The listing builds one solid part. Answer for the finished solid, in the listing's coordinates (mm). A direction names the side the tool comes from. Give positions to 0.01 mm unless a question says otherwise; leave off trailing zeros. Write each loop counter-clockwise with the first axis right and the second up, starting at its lowest first coordinate (ties: lowest second). Pieces come first, ordered by that corner, then holes. Notation, with made-up numbers: (70, -15.75) - (99, -15.75) arc R10 ccw to (99, 0.25) - close; hole circle Ø1 at (80, 60.25). An arc over 180 degrees is marked (long way). One line per item, written item: value. Start each with the question number.
Autodesk Inventor part; units mm, degrees
ref_plane "to_body_XY" through (0, 0, 0) normal (0, -1, 0) x (1, 0, 0)
ref_plane "to_body_YZ" through (0, 0, 0) normal (1, 0, 0) x (0, 0, 1)
ref_plane "to_body_ZX" through (0, 0, 0) normal (0, 0, 1) x (0, -1, 0)
sketch "Sketch_1" plane through (0, 0.508, 0) normal (0, 1, 0) x (1, 0, 0)
  line L0 (-4.445, 8.382) -> (-4.445, -8.382)
  line L1 (-4.445, -8.382) -> (4.445, -8.382)
  line L2 (4.445, -8.382) -> (4.445, 8.382)
  line L3 (4.445, 8.382) -> (-4.445, 8.382)
extrude "Extrusion1" add sketch "Sketch_1" against normal blind 0.254
sketch "Sketch_2" plane through (-2.4892, 0, 0) normal (1, 0, 0) x (0, 0, -1)
  line L0 (-7.3787, -7.62) -> (-6.9342, -8.255)
  line L1 (-6.9342, -8.255) -> (-3.0734, -8.255)
  line L2 (-3.0734, -8.255) -> (-2.6289, -7.62)
  line L3 (-2.6289, -7.62) -> (-2.6289, 0.508)
  line L4 (-2.6289, 0.508) -> (-7.3787, 0.508)
  line L5 (-7.3787, 0.508) -> (-7.3787, -7.62)
  arc A0 (-4.2207, -5.6252) -> (-5.7869, -5.6252) centre (-5.0038, -4.7752) ccw
  arc A1 (-5.7869, -5.6252) -> (-4.2207, -5.6252) centre (-5.0038, -5.461) ccw
extrude "Extrusion2" add sketch "Sketch_2" along normal mid plane 0.7874
sketch "Sketch_3" plane through (2.4892, 0, 0) normal (1, 0, 0) x (0, 0, -1)
  line L0 (-7.3787, -7.62) -> (-6.9342, -8.255)
  line L1 (-6.9342, -8.255) -> (-3.0734, -8.255)
  line L2 (-3.0734, -8.255) -> (-2.6289, -7.62)
  line L3 (-2.6289, -7.62) -> (-2.6289, 0.508)
  line L4 (-2.6289, 0.508) -> (-7.3787, 0.508)
  line L5 (-7.3787, 0.508) -> (-7.3787, -7.62)
  arc A0 (-4.2207, -5.6252) -> (-5.7869, -5.6252) centre (-5.0038, -4.7752) ccw
  arc A1 (-5.7869, -5.6252) -> (-4.2207, -5.6252) centre (-5.0038, -5.461) ccw
extrude "Extrusion3" add sketch "Sketch_3" along normal mid plane 0.7874
sketch "Sketch_4" plane through (-3.9878, 0, 0) normal (1, 0, 0) x (0, 0, -1)
  line L0 (0.9779, -0.3048) -> (0.9779, -1.016)
  line L1 (0.9779, -1.016) -> (1.6129, -1.016)
  line L2 (1.6129, -1.016) -> (1.6129, -7.62)
  line L3 (1.6129, -7.62) -> (2.0574, -8.255)
  line L4 (2.0574, -8.255) -> (5.9182, -8.255)
  line L5 (5.9182, -8.255) -> (6.3627, -7.62)
  line L6 (6.3627, -7.62) -> (6.3627, 0.508)
  line L7 (6.3627, 0.508) -> (1.6129, 0.508)
  line L8 (1.6129, 0.508) -> (1.6129, -0.3048)
  line L9 (1.6129, -0.3048) -> (0.9779, -0.3048)
  arc A0 (4.7709, -5.6252) -> (3.2047, -5.6252) centre (3.9878, -4.7752) ccw
  arc A1 (3.2047, -5.6252) -> (4.7709, -5.6252) centre (3.9878, -5.461) ccw
extrude "Extrusion4" add sketch "Sketch_4" along normal mid plane 0.7874
sketch "Sketch_5" plane through (3.9878, 0, 0) normal (1, 0, 0) x (0, 0, -1)
  line L0 (0.9779, -0.3048) -> (0.9779, -1.016)
  line L1 (0.9779, -1.016) -> (1.6129, -1.016)
  line L2 (1.6129, -1.016) -> (1.6129, -7.62)
  line L3 (1.6129, -7.62) -> (2.0574, -8.255)
  line L4 (2.0574, -8.255) -> (5.9182, -8.255)
  line L5 (5.9182, -8.255) -> (6.3627, -7.62)
  line L6 (6.3627, -7.62) -> (6.3627, 0.508)
  line L7 (6.3627, 0.508) -> (1.6129, 0.508)
  line L8 (1.6129, 0.508) -> (1.6129, -0.3048)
  line L9 (1.6129, -0.3048) -> (0.9779, -0.3048)
  arc A0 (4.7709, -5.6252) -> (3.2047, -5.6252) centre (3.9878, -4.7752) ccw
  arc A1 (3.2047, -5.6252) -> (4.7709, -5.6252) centre (3.9878, -5.461) ccw
extrude "Extrusion5" add sketch "Sketch_5" along normal mid plane 0.7874
sketch "Sketch_6" plane through (0, 0, 0) normal (0, 0, 1) x (1, 0, 0)
  line L0 (-5.08, -8.636) -> (5.08, -8.636)
  line L1 (5.08, -8.636) -> (5.08, 0)
  line L2 (5.08, 0) -> (4.3815, 0)
  line L3 (4.3815, 0) -> (4.3815, -7.62)
  line L4 (4.3815, -7.62) -> (4.2545, -8.255)
  line L5 (4.2545, -8.255) -> (3.7211, -8.255)
  line L6 (3.7211, -8.255) -> (3.5941, -7.62)
  line L7 (3.5941, -7.62) -> (3.5941, 0)
  line L8 (3.5941, 0) -> (2.8829, 0)
  line L9 (2.8829, 0) -> (2.8829, -7.62)
  line L10 (2.8829, -7.62) -> (2.7559, -8.255)
  line L11 (2.7559, -8.255) -> (2.2225, -8.255)
  line L12 (2.2225, -8.255) -> (2.0955, -7.62)
  line L13 (2.0955, -7.62) -> (2.0955, 0)
  line L14 (2.0955, 0) -> (-2.0955, 0)
  line L15 (-2.0955, 0) -> (-2.0955, -7.62)
  line L16 (-2.0955, -7.62) -> (-2.2225, -8.255)
  line L17 (-2.2225, -8.255) -> (-2.7559, -8.255)
  line L18 (-2.7559, -8.255) -> (-2.8829, -7.62)
  line L19 (-2.8829, -7.62) -> (-2.8829, 0)
  line L20 (-2.8829, 0) -> (-3.5941, 0)
  line L21 (-3.5941, 0) -> (-3.5941, -7.62)
  line L22 (-3.5941, -7.62) -> (-3.7211, -8.255)
  line L23 (-3.7211, -8.255) -> (-4.2545, -8.255)
  line L24 (-4.2545, -8.255) -> (-4.3815, -7.62)
  line L25 (-4.3815, -7.62) -> (-4.3815, 0)
  line L26 (-4.3815, 0) -> (-5.08, 0)
  line L27 (-5.08, 0) -> (-5.08, -8.636)
extrude "Extrusion6" cut sketch "Sketch_6" along normal mid plane 17.78
sketch "Sketch_8" plane through (0, 0, 0) normal (1, 0, 0) x (0, 1, 0)
  line L0 (0, 6.4198) -> (-1.1938, 6.4198)
  arc A0 (-1.1938, 6.4198) -> (-1.1938, 5.5054) centre (-1.1938, 5.9626) ccw
  line L1 (-1.1938, 5.5054) -> (0, 5.5054)
  line L2 (0, 5.5054) -> (0, 6.4198)
extrude "Extrusion7" cut sketch "Sketch_8" along normal mid plane 17.78
sketch "Sketch_9" plane through (0, 0, 0) normal (1, 0, 0) x (0, 1, 0)
  line L0 (0, 4.5021) -> (-1.1938, 4.5021)
  arc A0 (-1.1938, 4.5021) -> (-1.1938, 3.5877) centre (-1.1938, 4.0449) ccw
  line L1 (-1.1938, 3.5877) -> (0, 3.5877)
  line L2 (0, 3.5877) -> (0, 4.5021)
extrude "Extrusion8" cut sketch "Sketch_9" along normal mid plane 17.78
sketch "Sketch_10" plane through (0, 0, 0) normal (1, 0, 0) x (0, 1, 0)
  line L0 (0, -2.5718) -> (-1.1938, -2.5718)
  arc A0 (-1.1938, -2.5718) -> (-1.1938, -3.4862) centre (-1.1938, -3.029) ccw
  line L1 (-1.1938, -3.4862) -> (0, -3.4862)
  line L2 (0, -3.4862) -> (0, -2.5718)
extrude "Extrusion9" cut sketch "Sketch_10" along normal mid plane 17.78
sketch "Sketch_11" plane through (0, 0, 0) normal (1, 0, 0) x (0, 1, 0)
  line L0 (0, -4.4894) -> (-1.1938, -4.4894)
  arc A0 (-1.1938, -4.4894) -> (-1.1938, -5.4039) centre (-1.1938, -4.9466) ccw
  line L1 (-1.1938, -5.4039) -> (0, -5.4039)
  line L2 (0, -5.4039) -> (0, -4.4894)
extrude "Extrusion10" cut sketch "Sketch_11" along normal mid plane 17.78
ref_plane "to_body_XY" through (0, 0, 0) normal (0, -1, 0) x (1, 0, 0)
ref_plane "to_body_YZ" through (0, 0, 0) normal (1, 0, 0) x (0, 0, 1)
ref_plane "to_body_ZX" through (0, 0, 0) normal (0, 0, 1) x (0, -1, 0)
properties part number "CWSB2F-nonillumin_trmnls"
Item 1: Find section A-A on y = -6.75. Determine the outline of the cut face in (x, z).
Item 2: Straight lines are drawn through the part: line 1 along X through (y, z) = (-3, 4.25); line 2 along Y through (x, z) = (-4, -5) (3 decimals); line 3 along Y through (x, z) = (2.25, -3). For each, find the intervals that lie inside material, in ascending order.
Item 3: Each of these flat-tipped pins is pushed along its axis until it touches: pin 1 Ø0.9 at (x, y) = (4, -0.5) entering from +Z; pin 2 Ø3 at (y, z) = (-4.78, 5) entering from -X; pin 3 Ø0.9 at (x, y) = (2.5, -0.5) entering from +Z; pin 4 Ø1.5 at (x, y) = (0, -7) entering from -Z. Where does it stop, or does it pass through?
Item 4: Find section B-B on x = 2.5. Give the number of separate pieces and of enclosed holes in the cut face, plus the area to 3 significant figures.
Item 5: For faces 4 (the flat face through (2.096, -3.6, 5.6)), 5 (the flat face through (2.883, -3.6, 5.6)), 6 (the flat face through (-4.382, -3.6, -3)), determine the directions among +Z, -Z, +X, -X, +Y, -Y from which every point of the face is accessible in a straight line to the end or side of a thin tool.
Item 6: The mould has two halves that part along X. Classify faces 1 (the flat face through (0, 0.254, 0)), 2 (the flat face through (4.382, -3.6, -3)), 3 (the cylindrical face through (3.98, -3.62, -3.95)): +X half, -X half, draft (parallel to the pull), parting line (faces both ways), or undercut.
Values:
1. outline: (-4.38, -6.36) - (-3.59, -6.36) - (-3.59, -1.61) - (-4.38, -1.61) - close; (-2.88, 2.63) - (-2.1, 2.63) - (-2.1, 7.38) - (-2.88, 7.38) - close; (2.1, 2.63) - (2.88, 2.63) - (2.88, 7.38) - (2.1, 7.38) - close; (3.59, -6.36) - (4.38, -6.36) - (4.38, -1.61) - (3.59, -1.61) - close
2. line 1: -2.88 to -2.1, 2.1 to 2.88
2. line 2: -8.255 to -5.333, -4.217 to -1.648, 0 to 0.508
2. line 3: 0.25 to 0.51
3. pin 1: z = -0.98
3. pin 2: x = -2.88
3. pin 3: z = 7.38
3. pin 4: through
4. separate pieces: 1
4. enclosed holes: 3
4. area: 36.9 mm^2
5. face 4: +Z, -Z, -Y
5. face 5: +Z, -Z, +X, -Y
5. face 6: +Z, -Z, -X, -Y
6. face 1: undercut
6. face 2: +X half
6. face 3: draft
